```python
from build123d import *

# Parameters (mm, degrees)
SKETCH1_R                       = 19.05
BOSS_EXTRUDE1_DEPTH             = 4.826
M2_5_CLEARANCE_HOLE2_AT_2_COUNT = 2
M2_5_CLEARANCE_HOLE2_AT_2_PITCH = 6.096
CIRPATTERN1_COUNT               = 8


with BuildPart() as part:
    # Sketch1 → Boss-Extrude1 (new body)
    with BuildSketch(Plane(origin=(0, 0, 0), x_dir=(1, 0, 0), z_dir=(0, 1, 0))):
        Circle(SKETCH1_R)
    extrude(amount=BOSS_EXTRUDE1_DEPTH)

    # Sketch11 → M2.5 Clearance Hole2 (revolve, cut)
    with BuildSketch(Plane(origin=(0, 0, -15.875), x_dir=(0, 0, -1), z_dir=(1, 0, 0))):
        Polygon((0, 0), (0, 5.89269403), (1.35255, 5.08), (1.35255, 0), align=None)
    m2_5_clearance_hole2 = revolve(axis=Axis((0, -6.35, -15.875), (0, 1, 0)), mode=Mode.SUBTRACT)

    # M2.5 Clearance Hole2 at 2: M2.5 Clearance Hole2 ×2
    with Locations(*[(0, 0, i * M2_5_CLEARANCE_HOLE2_AT_2_PITCH) for i in range(1, M2_5_CLEARANCE_HOLE2_AT_2_COUNT)]):
        add(m2_5_clearance_hole2, mode=Mode.SUBTRACT)

    # CirPattern1: M2.5 Clearance Hole2 ×8 about axis
    cirpattern1_axis = Axis((0, 0, 0), (0, 1, 0))
    for i in range(1, CIRPATTERN1_COUNT):
        add(m2_5_clearance_hole2.rotate(cirpattern1_axis, i * 360 / CIRPATTERN1_COUNT), mode=Mode.SUBTRACT)

    # CirPattern1 copy 1 sketch → CirPattern1 copy 1 (revolve, cut)
    with BuildSketch(Plane(origin=(-6.914797213, 0, -6.914797213), x_dir=(-0.707106781, 0, -0.707106781), z_dir=(0.707106781, 0, -0.707106781))):
        Polygon((0, 0), (0, 5.89269403), (1.35255, 5.08), (1.35255, 0), align=None)
    revolve(axis=Axis((-6.914797213, -6.35, -6.914797213), (0, 1, 0)), mode=Mode.SUBTRACT)

    # CirPattern1 copy 2 sketch → CirPattern1 copy 2 (revolve, cut)
    with BuildSketch(Plane(origin=(-9.779, 0, 0), x_dir=(-1, 0, 0), z_dir=(0, 0, -1))):
        Polygon((0, 0), (0, 5.89269403), (1.35255, 5.08), (1.35255, 0), align=None)
    revolve(axis=Axis((-9.779, -6.35, 0), (0, 1, 0)), mode=Mode.SUBTRACT)

    # CirPattern1 copy 3 sketch → CirPattern1 copy 3 (revolve, cut)
    with BuildSketch(Plane(origin=(-6.914797213, 0, 6.914797213), x_dir=(-0.707106781, 0, 0.707106781), z_dir=(-0.707106781, 0, -0.707106781))):
        Polygon((0, 0), (0, 5.89269403), (1.35255, 5.08), (1.35255, 0), align=None)
    revolve(axis=Axis((-6.914797213, -6.35, 6.914797213), (0, 1, 0)), mode=Mode.SUBTRACT)

    # CirPattern1 copy 4 sketch → CirPattern1 copy 4 (revolve, cut)
    with BuildSketch(Plane(origin=(0, 0, 9.779), x_dir=(0, 0, 1), z_dir=(-1, 0, 0))):
        Polygon((0, 0), (0, 5.89269403), (1.35255, 5.08), (1.35255, 0), align=None)
    revolve(axis=Axis((0, -6.35, 9.779), (0, 1, 0)), mode=Mode.SUBTRACT)

    # CirPattern1 copy 5 sketch → CirPattern1 copy 5 (revolve, cut)
    with BuildSketch(Plane(origin=(6.914797213, 0, 6.914797213), x_dir=(0.707106781, 0, 0.707106781), z_dir=(-0.707106781, 0, 0.707106781))):
        Polygon((0, 0), (0, 5.89269403), (1.35255, 5.08), (1.35255, 0), align=None)
    revolve(axis=Axis((6.914797213, -6.35, 6.914797213), (0, 1, 0)), mode=Mode.SUBTRACT)

    # CirPattern1 copy 6 sketch → CirPattern1 copy 6 (revolve, cut)
    with BuildSketch(Plane(origin=(9.779, 0, 0), x_dir=(1, 0, 0), z_dir=(0, 0, 1))):
        Polygon((0, 0), (0, 5.89269403), (1.35255, 5.08), (1.35255, 0), align=None)
    revolve(axis=Axis((9.779, -6.35, 0), (0, 1, 0)), mode=Mode.SUBTRACT)

    # CirPattern1 copy 7 sketch → CirPattern1 copy 7 (revolve, cut)
    with BuildSketch(Plane(origin=(6.914797213, 0, -6.914797213), x_dir=(0.707106781, 0, -0.707106781), z_dir=(0.707106781, 0, 0.707106781))):
        Polygon((0, 0), (0, 5.89269403), (1.35255, 5.08), (1.35255, 0), align=None)
    revolve(axis=Axis((6.914797213, -6.35, -6.914797213), (0, 1, 0)), mode=Mode.SUBTRACT)


solid = part.part
```
Geometry check sheet. Reference: the model listing, model coordinates, mm. Coordinates: 2 decimals unless noted, no trailing zeros. Loops run counter-clockwise (first coordinate to the right, second up) from the corner with the lowest first, then second, coordinate; pieces in that order, holes last.
Item 1: Thickness scan on line 1 (Z direction, x = 0, y = 1.45); line 2 (Z direction, x = -11, y = 3.5); line 3 (Z direction, x = -6.5, y = 0.7). Record the ranges inside material, lowest first.
Item 2: Go/stop test with flat-tipped pins: pin 1 Ø2 at (x, y) = (-11, 1.5) entering from +Z; pin 2 Ø1.5 at (x, z) = (6.5, 7) entering from -Y; pin 3 Ø2 at (x, y) = (9, 1) entering from -Z. Record where each tip stops, or that it passes through.
Item 3: Release check for a two-part mould opening along X. For faces 1 (the face through (0, 4.826, 0)), 2 (the face through (-6.738, 2.379, 5.574)), 3 (the face through (-15.12, 2.38, 11.59)) record: released by +X, released by -X, zero draft, split by the parting line, or undercut.
Item 4: Sectioned sample at D-D, the plane y = 4.1. Count the separate pieces of the cut face and the enclosed holes in it, then the cut area to 3 significant figures.
Item 5: Sectioned sample at B-B, the plane x = -9. Record the boundary of the cut face in (y, z).
Item 6: Sectioned sample at A-A, the plane z = 0. Record the boundary of the cut face in (x, y).
Item 7: Sectioned sample at C-C, the plane x = 0. Record the boundary of the cut face in (y, z).
Check result:
1. line 1: z = -19.05 to -17.23, -14.52 to -11.13, -8.43 to 8.43, 11.13 to 14.52, 17.23 to 19.05
1. line 2: z = -15.55 to -12.56, -9.89 to -0.58, 0.58 to 9.89, 12.56 to 15.55
1. line 3: z = -17.91 to -8.2, -5.63 to 5.63, 8.2 to 17.91
2. pin 1: stops at z = 16.21
2. pin 2: passes through
2. pin 3: stops at z = -17.29
3. face 1: zero draft
3. face 2: undercut
3. face 3: split by the parting line
4. separate pieces: 1
4. enclosed holes: 16
4. area: 1,050 mm2
5. outline: (0, -16.79) - (4.83, -16.79) - (4.83, -1.11) - (0, -1.11) - close; (0, 1.11) - (4.83, 1.11) - (4.83, 16.79) - (0, 16.79) - close
6. outline: (-19.05, 0) - (-17.23, 0) - (-17.23, 4.83) - (-19.05, 4.83) - close; (-14.52, 0) - (-11.13, 0) - (-11.13, 4.83) - (-14.52, 4.83) - close; (-8.43, 0) - (8.43, 0) - (8.43, 4.83) - (-8.43, 4.83) - close; (11.13, 0) - (14.52, 0) - (14.52, 4.83) - (11.13, 4.83) - close; (17.23, 0) - (19.05, 0) - (19.05, 4.83) - (17.23, 4.83) - close
7. outline: (0, -19.05) - (4.83, -19.05) - (4.83, -17.23) - (0, -17.23) - close; (0, -14.52) - (4.83, -14.52) - (4.83, -11.13) - (0, -11.13) - close; (0, -8.43) - (4.83, -8.43) - (4.83, 8.43) - (0, 8.43) - close; (0, 11.13) - (4.83, 11.13) - (4.83, 14.52) - (0, 14.52) - close; (0, 17.23) - (4.83, 17.23) - (4.83, 19.05) - (0, 19.05) - close
